Geometry check sheet. Reference: the model listing, model coordinates, mm. Round coordinates to 2 decimals unless told otherwise and drop trailing zeros. Write each loop counter-clockwise with the first axis right and the second up, starting at its lowest first coordinate (ties: lowest second). Pieces come first, ordered by that corner, then holes. Notation, with made-up numbers: (81.5, 47) - (100.5, 47) arc R20 cw to (100.5, 79) - close; hole circle Ø2 at (66, -21). An arc over 180 degrees is marked (long way). Return JSON: item names as keys, results as strings. Group by question number.
from build123d import *

# Parameters (mm, degrees)
F1_DEPTH  = 250
F0_W      = 10
F0_H      = 75
F2_DEPTH  = 25
F3_R      = 5
F4_DEPTH  = 380.001
F5_R      = 5
F6_W      = 25
F6_H      = 350
F7_DEPTH  = 25
F8_W      = 10
F8_H      = 25
F9_DEPTH  = 50
F10_R     = 5
F11_DEPTH = 380.001


with BuildPart() as f1:
    # F0 (on Front) → F1 (new body)
    with BuildSketch(Plane.XZ):
        Polygon((-268.93918, 1.907515), (-278.93918, 1.907515), (-278.93918, -8.092485), (101.06082, -8.092485), (101.06082, 1.907515), (91.06082, 1.907515), align=None)
    extrude(amount=F1_DEPTH)

    # F0 (on Front) → F2 (join)
    with BuildSketch(Plane.XZ):
        with Locations((-273.93918, 39.407515)):
            Rectangle(F0_W, F0_H)
        Polygon((-268.93918, 1.907515), (-278.93918, 1.907515), (-278.93918, -8.092485), (101.06082, -8.092485), (101.06082, 1.907515), (91.06082, 1.907515), align=None)
        with Locations((96.06082, 39.407515)):
            Rectangle(F0_W, F0_H)
    extrude(amount=F2_DEPTH)

    # F3 (on face) → F4 (cut, through all)
    with BuildSketch(Plane(origin=(-278.93918, 0, 0), x_dir=(0, -1, 0), z_dir=(-1, 0, 0))):
        with Locations((11.970147, 61.907515)):
            Circle(F3_R)
    extrude(amount=-F4_DEPTH, mode=Mode.SUBTRACT)

    # F5
    f5_edges = [f1.edges().sort_by_distance(p)[0] for p in [
        (-273.93918, 0, 76.907515),
        (-273.93918, -25, 76.907515),
        (96.06082, 0, 76.907515),
        (96.06082, -25, 76.907515),
    ]]
    fillet(f5_edges, radius=F5_R)

    # F6 (on face) → F7 (join)
    with BuildSketch(Plane.XY.offset(1.907515)):
        with Locations((88.56082, -175)):
            Rectangle(F6_W, F6_H)
    extrude(amount=F7_DEPTH)

    # F8 (on face) → F9 (join)
    with BuildSketch(Plane.XY.offset(26.907515)):
        with Locations((96.06082, -323.5)):
            Rectangle(F8_W, F8_H)
    extrude(amount=F9_DEPTH)

    # F10 (on face) → F11 (cut, through all)
    with BuildSketch(Plane.YZ.offset(101.06082)):
        with Locations((-323.5, 60.567401)):
            Circle(F10_R)
    extrude(amount=-F11_DEPTH, mode=Mode.SUBTRACT)


solid = f1.part
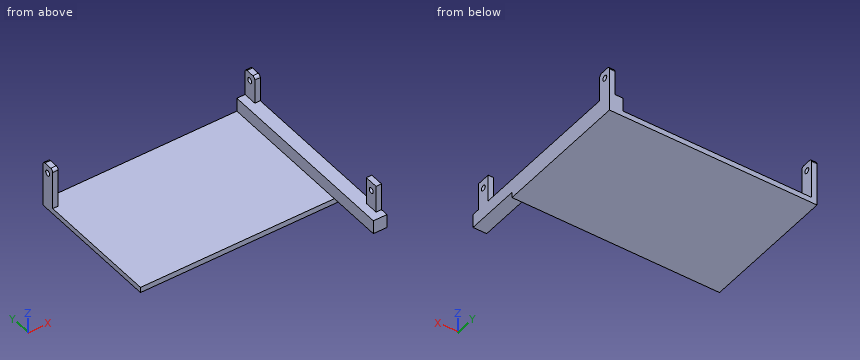
1. Depth check by flat-ended pin: pin 1 Ø3 at (x, z) = (97, 43) entering from -Y; pin 2 Ø9 at (y, z) = (-323.5, 60.57) entering from +X; pin 3 Ø3 at (x, z) = (-274.5, 25) entering from -Y; pin 4 Ø12.5 at (y, z) = (-325, 46.5) entering from -X. Enter the tip coordinate at first touch or a pass-through.
2. Section check A-A (z = 19). Enter the section's corners in (x, y), and give its area (3 significant figures).
3. Section check C-C (z = 49). Enter the section's corners in (x, y), and give its area (3 significant figures).
4. Section check D-D (x = -187). Enter the section's corners in (y, z), and give its area (3 significant figures).
5. Material ranges on line 1 along Z through (x, y) = (94.5, -323.5); line 2 along Z through (x, y) = (0.5, -79); line 3 along X through (y, z) = (-268, 4), recorded low to high.
6. Section check B-B (y = -323.5). Enter the section's corners in (x, z), and give its area (4 significant figures).
Result sheet:
{
 "1": {"pin 1": "stops at y = -336", "pin 2": "passes through", "pin 3": "stops at y = -25", "pin 4": "stops at x = 91.06"},
 "2": {"outline": "(-278.94, -25) - (-268.94, -25) - (-268.94, 0) - (-278.94, 0) - close; (76.06, -350) - (101.06, -350) - (101.06, 0) - (76.06, 0) - close", "area": "9,000 mm²"},
 "3": {"outline": "(-278.94, -25) - (-268.94, -25) - (-268.94, 0) - (-278.94, 0) - close; (91.06, -336) - (101.06, -336) - (101.06, -311) - (91.06, -311) - close; (91.06, -25) - (101.06, -25) - (101.06, 0) - (91.06, 0) - close", "area": "750 mm²"},
 "4": {"outline": "(-250, -8.09) - (0, -8.09) - (0, 1.91) - (-250, 1.91) - close", "area": "2,500 mm²"},
 "5": {"line 1": "z = 1.91 to 55.57, 65.57 to 76.91", "line 2": "z = -8.09 to 1.91", "line 3": "x = 76.06 to 101.06"},
 "6": {"outline": "(76.06, 1.91) - (101.06, 1.91) - (101.06, 55.57) - (91.06, 55.57) - (91.06, 26.91) - (76.06, 26.91) - close; (91.06, 65.57) - (101.06, 65.57) - (101.06, 76.91) - (91.06, 76.91) - close", "area": "1,025 mm²"}
}
